Input: dimensioned drawing with shaded views. Units: mm. Origin: part minimum x, y, z. Round coordinates to 2 decimals unless told otherwise and drop trailing zeros. Loops run counter-clockwise (first coordinate to the right, second up) from the corner with the lowest first, then second, coordinate; pieces in that order, holes last. Notation, with made-up numbers: M 2,27.25 L 11,27.25 A13 cw 11,51.25 Z; hole C 85.25,27.25 d11. An arc over 180 degrees is marked long. Answer as CSV lines item,"result". Start each with the question number.
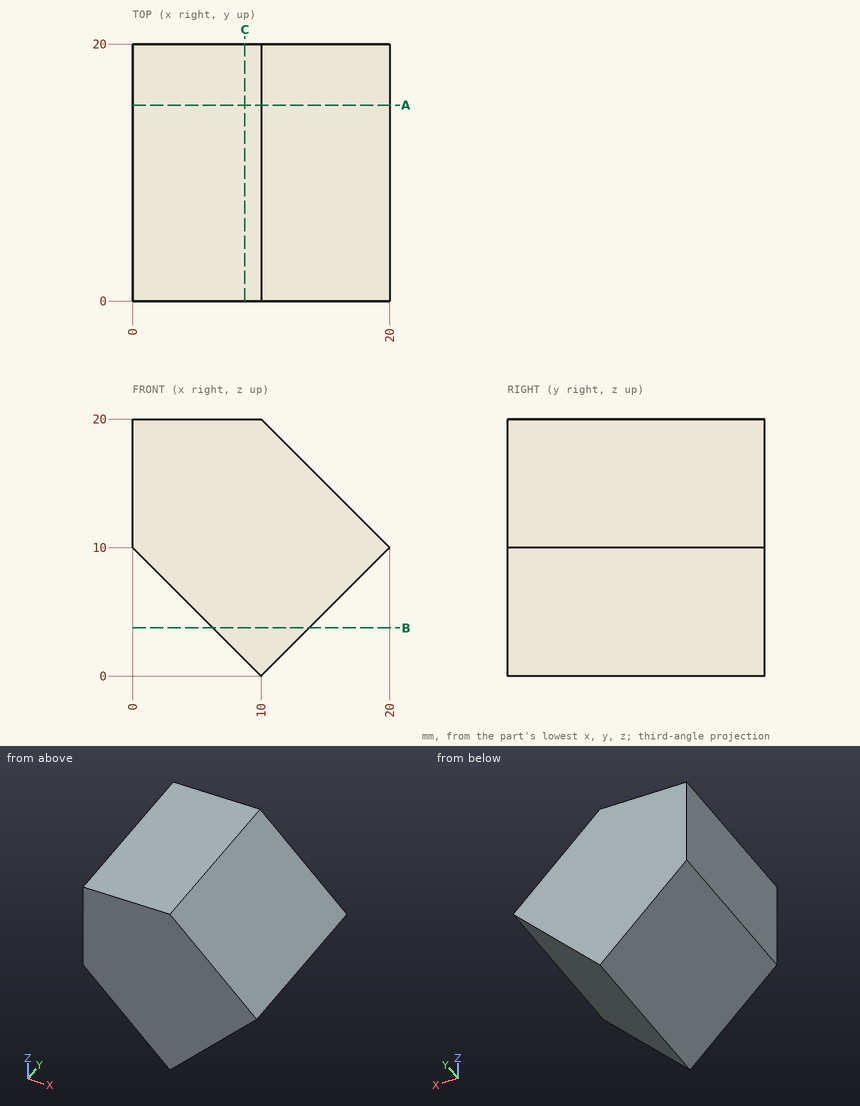
1) Ray query, line 1 along X through (y, z) = (1.5, 17.25); line 2 along X through (y, z) = (16, 1.75); line 3 along Z through (x, y) = (3.25, 14). Return the intervals inside material, ascending.
2) Contact query for flat-ended pins moving along their axis: pin 1 Ø1 at (y, z) = (14.5, 2) entering from +X; pin 2 Ø5 at (y, z) = (7.5, 13.5) entering from +X; pin 3 Ø1.5 at (y, z) = (13, 9.5) entering from +X. Output: stop coordinate, or through.
3) Section B-B, the plane z = 3.75. Return loops of the section in (x, y), and give its area (3 significant figures).
4) Section A-A, the plane y = 15.25. Return loops of the section in (x, z).
5) Section C-C, the plane x = 8.75. Return loops of the section in (y, z), and give its area (3 significant figures).
Findings below:
1,line 1,"0 to 12.75"
1,line 2,"8.25 to 11.75"
1,line 3,"6.75 to 20"
2,pin 1,"x = 12.5"
2,pin 2,"x = 19"
2,pin 3,"x = 20"
3,outline,"M 6.25,0 L 13.75,0 L 13.75,20 L 6.25,20 Z"
3,area,"150 mm²"
4,outline,"M 0,10 L 10,0 L 20,10 L 10,20 L 0,20 Z"
5,outline,"M 0,1.25 L 20,1.25 L 20,20 L 0,20 Z"
5,area,"375 mm²"
